Could you check a few things on this drawing? It's one solid part, dimensions in mm from its lowest x, y, z. A direction names the side the tool comes from. Give positions to 0.01 mm unless a question says otherwise; leave off trailing zeros. Order: outer loops, then holes, each group sorted by start corner. A loop starts at its lowest first (then second) coordinate and runs counter-clockwise, first axis right, second up.
Item 1: I want a section at B-B, the plane x = 11. Write out the boundary of the cut face in (y, z), then the cut area to 3 significant figures.
Item 2: If I drill on line 1 along Z through (x, y) = (10, 13); line 2 along Y through (x, z) = (2.5, 60); line 3 along Z through (x, y) = (39.5, 104), over which ranges is the centre line in solid material (lowest first)?
Item 3: I want a section at C-C, the plane z = 81. Write out the boundary of the cut face in (x, y).
Item 4: I want a section at A-A, the plane y = 86.7. Write out the boundary of the cut face in (x, z), then the cut area to 3 significant figures.
Item 5: I want a section at D-D, the plane y = 58. Write out the boundary of the cut face in (x, z), then the cut area to 3 significant figures.
Item 6: I'm going to push flat-ended pins straight in: pin 1 Ø2 at (x, y) = (12, 51) entering from -Z; pin 2 Ø4.5 at (y, z) = (92, 88) entering from +X; pin 3 Ø12 at (x, y) = (7.5, 169.5) entering from +Z; pin 4 Ø3.5 at (x, y) = (22.1, 86.7) entering from -Z. Where does each tip first touch, or does it pass through?
Item 7: Which directions (+Z, -Z, +X, -X, +Y, -Y) give clear straight access to the entire face, cutting with the end or side of a thin tool? Please do the marked faces 1, 2, 3, 4 and 5.
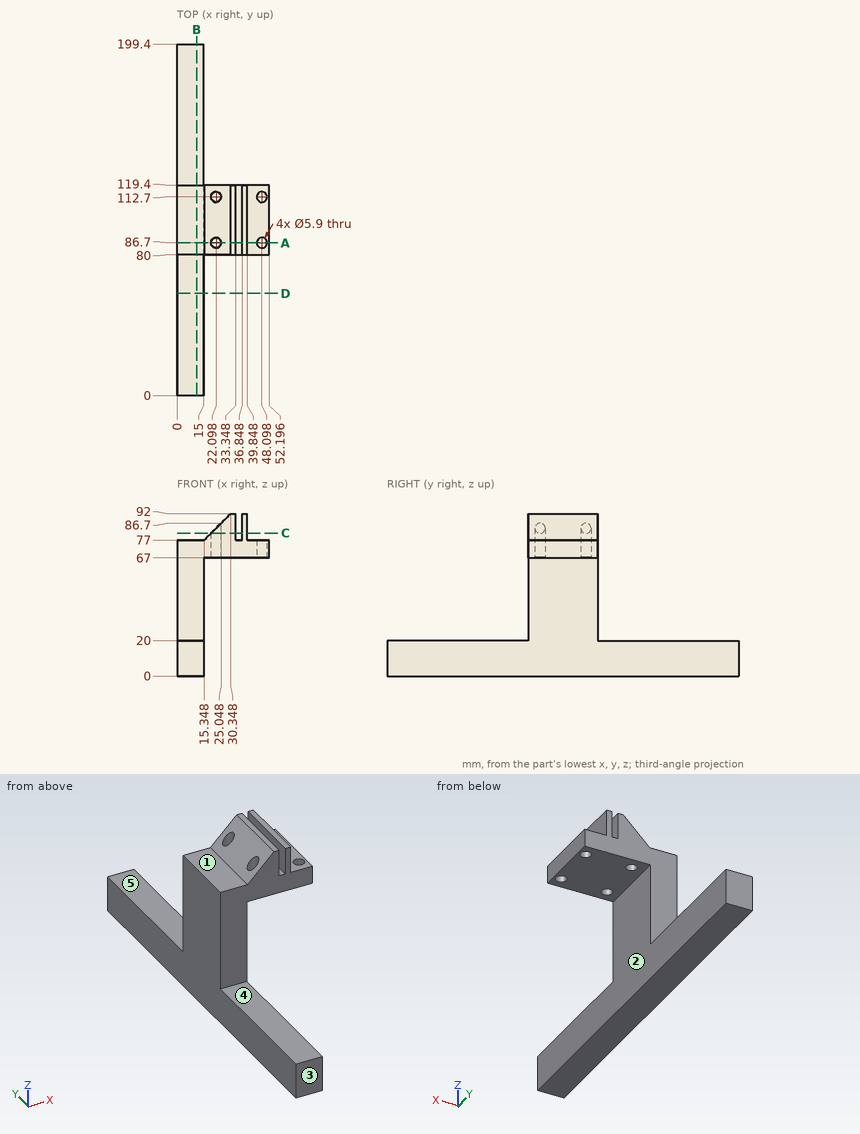
Results list:
1. outline: (0, 0) - (199.4, 0) - (199.4, 20) - (119.4, 20) - (119.4, 77) - (80, 77) - (80, 20) - (0, 20) - close
1. area: 6,230 mm2
2. line 1: z = 0 to 20
2. line 2: y = 80 to 119.4
2. line 3: z = 67 to 92
3. outline: (19.35, 80) - (33.35, 80) - (33.35, 119.4) - (19.35, 119.4) - (19.35, 113.77) arc R2.95 cw (long way) to (19.35, 111.63) - (19.35, 87.77) arc R2.95 cw (long way) to (19.35, 85.63) - close; (36.85, 80) - (39.85, 80) - (39.85, 119.4) - (36.85, 119.4) - close
4. outline: (0, 0) - (15, 0) - (15, 67) - (19.15, 67) - (19.15, 80.8) - (15.35, 77) - (0, 77) - close; (25.05, 67) - (45.15, 67) - (45.15, 77) - (39.85, 77) - (39.85, 92) - (36.85, 92) - (36.85, 77) - (33.35, 77) - (33.35, 92) - (30.35, 92) - (25.05, 86.7) - close; (51.05, 67) - (52.2, 67) - (52.2, 77) - (51.05, 77) - close
4. area: 1,570 mm2
5. outline: (0, 0) - (15, 0) - (15, 20) - (0, 20) - close
5. area: 300 mm2
6. pin 1: stops at z = 0
6. pin 2: stops at x = 39.85
6. pin 3: stops at z = 20
6. pin 4: passes through
7. face 1: +Z, -X, +Y, -Y
7. face 2: -Z, +X, +Y, -Y
7. face 3: +Z, -Z, +X, -X, -Y
7. face 4: +Z, +X, -X, -Y
7. face 5: +Z, +X, -X, +Y
